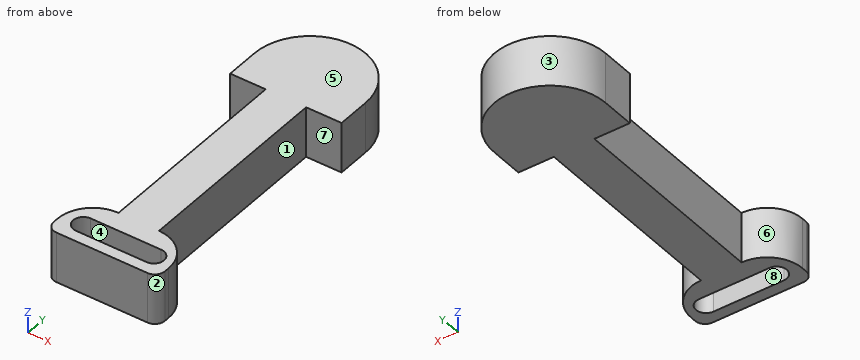
from build123d import *

# Parameters (mm, degrees)
F0_W     = 101.6
F0_H     = 508
F1_DEPTH = 127
F2_R     = 88.89999
F3_R     = 88.89999
F5_DEPTH = 127.001
F6_R     = 25.4
F7_R     = 25.4


# Not quite as in the source:
# - a fillet or chamfer is up to 0.001 mm smaller than in the source, because OpenCascade refuses the exact size


with BuildPart() as f1:
    # F0 (on Top) → F1 (new body)
    with BuildSketch(Plane.XY):
        with BuildLine():
            ThreePointArc((139.7, 83.3142390684), (0, 223.0142390684), (-139.7, 83.3142390684))
            Line((-139.7, 83.3142390684), (-139.7, 0))
            Line((-139.7, 0), (-50.8, 0))
            Line((-50.8, 0), (50.8, 0))
            Line((50.8, 0), (139.7, 0))
            Line((139.7, 0), (139.7, 83.3142390684))
        make_face()
        with Locations((0, -254)):
            Rectangle(F0_W, F0_H)
        Polygon((50.8, -508), (-50.8, -508), (-139.7, -508), (-139.7, -635), (139.7, -635), (139.7, -508), align=None)
    extrude(amount=F1_DEPTH)

    # F2 (radius 88.9 in the source; OpenCascade refuses exactly that, so slightly less here)
    f2_edges = [f1.edges().sort_by_distance(p)[0] for p in [
        (139.7, -508, 63.5),
    ]]
    fillet(f2_edges, radius=F2_R)

    # F3 (radius 88.9 in the source; OpenCascade refuses exactly that, so slightly less here)
    f3_edges = [f1.edges().sort_by_distance(p)[0] for p in [
        (-139.7, -508, 63.5),
    ]]
    fillet(f3_edges, radius=F3_R)

    # F4 (on face) → F5 (cut, through all)
    with BuildSketch(Plane.XY.offset(127)):
        with BuildLine():
            Line((91.3110496293, -556.0355413279), (-85.6204037596, -556.0355413279))
            ThreePointArc((-85.6204037596, -556.0355413279), (-111.0204037596, -581.4355413279), (-85.6204037596, -606.8355413279))
            Line((-85.6204037596, -606.8355413279), (91.3110496293, -606.8355413279))
            ThreePointArc((91.3110496293, -606.8355413279), (116.7110496293, -581.4355413279), (91.3110496293, -556.0355413279))
        make_face()
    extrude(amount=-F5_DEPTH, mode=Mode.SUBTRACT)

    # F6
    f6_edges = [f1.edges().sort_by_distance(p)[0] for p in [
        (139.7, -635, 63.5),
    ]]
    fillet(f6_edges, radius=F6_R)

    # F7
    f7_edges = [f1.edges().sort_by_distance(p)[0] for p in [
        (-139.7, -635, 63.5),
    ]]
    fillet(f7_edges, radius=F7_R)


solid = f1.part
The model under review builds one solid part; all positions refer to its coordinate system, in mm. Face numbers are marked on the shaded views. A direction names the side the tool comes from. Give positions to 0.01 mm unless a question says otherwise; leave off trailing zeros. Write each loop counter-clockwise with the first axis right and the second up, starting at its lowest first coordinate (ties: lowest second). Pieces come first, ordered by that corner, then holes.
1. For P1, Ø8, axis at y = -513, z = 72, coming from the -X side; P2, Ø1.5, axis at y = -18, z = 71.5, coming from the -X side; P3, Ø10, axis at y = -101.5, z = 84.5, coming from the +X side, all flat-tipped, find the tip position at first contact; note any pin that passes through.
2. Tool access review of the marked faces 5, 6, 7 and 8: name each direction out of +Z, -Z, +X, -X, +Y, -Y from which nothing blocks a thin tool from reaching the whole face with its end or side.
3. Add section D-D, the plane y = -458. Write out the cut boundary in (x, z).
4. Draft analysis for pull direction Y (two halves, no side actions). For the marked faces 1, 2, 3 and 4, state which applies: +Y half, -Y half, draft (parallel to the pull), parting line (faces both ways), or undercut.
5. Wall thickness on L1, parallel to Y at x = -76.5, z = 69; L2, parallel to Y at x = 95, z = 92; L3, parallel to X at y = -500.5, z = 102.5: over which ranges is each line inside the solid? List them lowest first.
6. Add section C-C, the plane x = -77. Write out the cut boundary in (y, z).
7. Add section A-A, the plane x = 0. Write out the cut boundary in (y, z).
Worked answers:
1. P1: stops at x = -89.78
1. P2: stops at x = -50.8
1. P3: stops at x = 50.8
2. face 5: +Z, +X, -X, +Y, -Y
2. face 6: +Z, -Z, -X
2. face 7: +Z, -Z, +X
2. face 8: +Z, -Z
3. outline: (-50.8, 0) - (50.8, 0) - (50.8, 127) - (-50.8, 127) - close
4. face 1: undercut
4. face 2: -Y half
4. face 3: +Y half
4. face 4: undercut
5. L1: y = -635 to -606.84, -556.04 to -511.8, 0 to 200.21
5. L2: y = -635 to -606.57, -556.3 to -519.77, 0 to 185.74
5. L3: x = -50.8 to 50.8
6. outline: (-635, 0) - (-606.84, 0) - (-606.84, 127) - (-635, 127) - close; (-556.04, 0) - (-511.95, 0) - (-511.95, 127) - (-556.04, 127) - close; (0, 0) - (199.88, 0) - (199.88, 127) - (0, 127) - close
7. outline: (-635, 0) - (-606.84, 0) - (-606.84, 127) - (-635, 127) - close; (-556.04, 0) - (223.01, 0) - (223.01, 127) - (-556.04, 127) - close
